from build123d import *

# Parameters (mm, degrees)
ESTRUSIONE_ESTRUSIONE8_DEPTH = 5
SCHIZZO19_W                  = 5
SCHIZZO19_H                  = 46.212351189
ESTRUSIONE_ESTRUSIONE9_DEPTH = 6.5
SCHIZZO20_R                  = 1.75
TAGLIO_ESTRUSIONE9_DEPTH     = 6
TAGLIO_ESTRUSIONE13_DEPTH    = 21
SCHIZZO26_W                  = 5
SCHIZZO26_H                  = 6.5
TAGLIO_ESTRUSIONE15_DEPTH    = 21
RACCORDO1_R                  = 10
SMUSSO1_SIZE                 = 12


with BuildPart() as part:
    # Schizzo18 → Estrusione-Estrusione8 (new body)
    with BuildSketch(Plane(origin=(0, 40, 0), x_dir=(1, 0, 0), z_dir=(0, 1, 0))):
        Polygon((25, -16), (-9, -16), (-9, 30.212351189), (-4.036856652, 30.212351189), (5.487873038, 7), (25, 7), align=None)
        with BuildLine():
            Line((17.25, -11), (17.25, -7))
            ThreePointArc((17.25, -7), (19, -5.25), (20.75, -7))
            Line((20.75, -7), (20.75, -11))
            ThreePointArc((20.75, -11), (19, -12.75), (17.25, -11))
        make_face(mode=Mode.SUBTRACT)
        with BuildLine():
            Line((7.74056589, -11), (7.74056589, -7))
            ThreePointArc((7.74056589, -7), (9.49056589, -5.25), (11.24056589, -7))
            Line((11.24056589, -7), (11.24056589, -11))
            ThreePointArc((11.24056589, -11), (9.49056589, -12.75), (7.74056589, -11))
        make_face(mode=Mode.SUBTRACT)
    extrude(amount=ESTRUSIONE_ESTRUSIONE8_DEPTH)

    # Schizzo19 → Estrusione-Estrusione9 (add)
    with BuildSketch(Plane.XZ.offset(-40)):
        with Locations((-6.5, -7.106175595)):
            Rectangle(SCHIZZO19_W, SCHIZZO19_H)
    extrude(amount=ESTRUSIONE_ESTRUSIONE9_DEPTH)

    # Schizzo20 → Taglio-Estrusione9 (cut)
    with BuildSketch(Plane.ZY.offset(9)):
        with Locations((-24, 36.5)):
            Circle(SCHIZZO20_R)
        with Locations((-14, 36.5)):
            Circle(SCHIZZO20_R)
    extrude(amount=-TAGLIO_ESTRUSIONE9_DEPTH, mode=Mode.SUBTRACT)

    # Schizzo24 → Taglio-Estrusione13 (cut)
    with BuildSketch(Plane(origin=(0, 45, 0), x_dir=(1, 0, 0), z_dir=(0, 1, 0))):
        Polygon((3.042265575, -16), (-9, 7.106175595), (-9, -16), align=None)
    extrude(amount=-TAGLIO_ESTRUSIONE13_DEPTH, mode=Mode.SUBTRACT)

    # Schizzo26 → Taglio-Estrusione15 (cut)
    with BuildSketch(Plane.XY.offset(-7.106175595)):
        with Locations((-6.5, 36.75)):
            Rectangle(SCHIZZO26_W, SCHIZZO26_H)
    extrude(amount=TAGLIO_ESTRUSIONE15_DEPTH, mode=Mode.SUBTRACT)

    # Raccordo1
    raccordo1_edges = [part.edges().sort_by_distance(p)[0] for p in [
        (3.042265575, 42.5, 16),
    ]]
    fillet(raccordo1_edges, radius=RACCORDO1_R)

    # Smusso1
    smusso1_edges = [part.edges().sort_by_distance(p)[0] for p in [
        (25, 42.5, -7),
    ]]
    chamfer(smusso1_edges, length=SMUSSO1_SIZE)


solid = part.part
The listing builds one solid part. Answer for the finished solid, in the listing's coordinates (mm). A direction names the side the tool comes from. Coordinates: 2 decimals unless noted, no trailing zeros. Loops run counter-clockwise (first coordinate to the right, second up) from the corner with the lowest first, then second, coordinate; pieces in that order, holes last. Notation, with made-up numbers: (82.25, 51) -> (141.25, 51) arc R15 ccw to (141.25, 64) -> close; hole circle Ø1 at (66, 37.5). An arc over 180 degrees is marked (long way). Write item = value, one per line. Start each with the question number.
1) A cutting plane is placed at D-D (y = 42.5). Give the vertices of the cut face in (x, z).
2) A cutting plane is placed at B-B (y = 36.5). Give the vertices of the cut face in (x, z), then the cut area to 3 significant figures.
3) A tool of negligible diameter and unlimited length cuts with its end or side. For faces 4 (the face through (9, 42, -7)), 5 (the face through (-6.54, 34.95, -13.19)), 6 (the face through (7.741, 42, 9)), 7 (the face through (-4, 37, -19)), from which of +Z, -Z, +X, -X, +Y, -Y can it reach the whole face along a straight path? Write none if from no direction.
4) Given pin 1 Ø1.5 at (x, y) = (0.5, 37.5) entering from -Z; pin 2 Ø4.5 at (y, z) = (36.5, -24) entering from +X; pin 3 Ø1.5 at (x, y) = (10, 42) entering from -Z; pin 4 Ø4.5 at (y, z) = (42.5, 9.5) entering from -X, each flat-ended and moving along its own axis, determine where each tip first touches the part or whether it passes through.
5) A cutting plane is placed at A-A (x = 19). Give the vertices of the cut face in (y, z), then the cut area to 3 significant figures.
6) A cutting plane is placed at C-C (z = -14). Give the vertices of the cut face in (x, y), then the cut area to 3 significant figures.
7) Straight lines are drawn through the part: line 1 (Y direction, x = -7.7, z = -24); line 2 (X direction, y = 40.5, z = 7); line 3 (X direction, y = 39, z = -19.5). For each, find the intervals that lie inside material, in ascending order. Write a range as from..to.
8) The mould has two halves that part along X. Classify faces 1 (the face through (0.66, 42.46, -18.77)), 2 (the face through (-7, 37, -7.106)), 3 (the face through (9.53, 42.46, 12.75)): released by +X, released by -X, zero draft, split by the parting line, or undercut.
Responses:
q1.outline = (-9, -30.21) -> (-4.04, -30.21) -> (5.49, -7) -> (13, -7) -> (25, 5) -> (25, 16) -> (9.11, 16) arc R10 ccw to (0.24, 10.62) -> (-9, -7.11) -> close; hole (7.74, 7) arc R1.75 ccw to (11.24, 7) -> (11.24, 11) arc R1.75 ccw to (7.74, 11) -> close; hole (17.25, 7) arc R1.75 ccw to (20.75, 7) -> (20.75, 11) arc R1.75 ccw to (17.25, 11) -> close
q2.outline = (-9, -30.21) -> (-4, -30.21) -> (-4, -25.75) -> (-9, -25.75) -> close; (-9, -22.25) -> (-4, -22.25) -> (-4, -15.75) -> (-9, -15.75) -> close; (-9, -12.25) -> (-4, -12.25) -> (-4, -7.11) -> (-9, -7.11) -> close
q2.area = 80.5 mm²
q3.face_4 = -Z, +X, +Y, -Y
q3.face_5 = +X, -X
q3.face_6 = +Y, -Y
q3.face_7 = +Z, -Z, +X, -Y
q4.pin_1 = through
q4.pin_2 = -4
q4.pin_3 = -7
q4.pin_4 = -1.52
q5.outline = (40, -1) -> (45, -1) -> (45, 5.25) -> (40, 5.25) -> close; (40, 12.75) -> (45, 12.75) -> (45, 16) -> (40, 16) -> close
q5.area = 47.5 mm²
q6.outline = (-9, 33.5) -> (-4, 33.5) -> (-4, 34.75) -> (-9, 34.75) -> close; (-9, 38.25) -> (-4, 38.25) -> (-4, 40) -> (2.62, 40) -> (2.62, 45) -> (-9, 45) -> close
q6.area = 73.1 mm²
q7.line_1 = 33.5..34.75, 38.25..45
q7.line_2 = -1.65..7.74, 11.24..17.25, 20.75..25
q7.line_3 = -9..-4
q8.face_1 = released by +X
q8.face_2 = zero draft
q8.face_3 = undercut
